from build123d import *

# Parameters (mm, degrees)
SKETCH1_W               = 8
SKETCH1_H               = 8
BOSS_EXTRUDE1_DEPTH     = 3
CUT_EXTRUDE1_DEPTH      = 12.704699911
CUT_EXTRUDE1_DEPTH_BACK = 12.704699911
CUT_EXTRUDE2_DEPTH      = 11
SKETCH4_R               = 1.8
CUT_EXTRUDE3_DEPTH      = 0.8
SKETCH5_W               = 8
SKETCH5_H               = 1
BOSS_EXTRUDE2_DEPTH     = 2
FILLET1_R               = 4
SKETCH6_W               = 0.769230769
SKETCH6_H               = 4
CUT_EXTRUDE4_DEPTH      = 0.4


with BuildPart() as part:
    # Sketch1 → Boss-Extrude1 (new body)
    with BuildSketch(Plane(origin=(0, 0, 0), x_dir=(1, 0, 0), z_dir=(0, 1, 0))):
        with Locations((4, 4)):
            Rectangle(SKETCH1_W, SKETCH1_H)
    extrude(amount=BOSS_EXTRUDE1_DEPTH)

    # Sketch2 → Cut-Extrude1 (cut, two sides: drawn at the far end of the back side and taken through both)
    with BuildSketch(Plane.XY.offset(-CUT_EXTRUDE1_DEPTH_BACK)):
        Polygon((0, 0), (0.6, 3), (0, 3), align=None)
        Polygon((8, 0), (7.4, 3), (8, 3), align=None)
    extrude(amount=CUT_EXTRUDE1_DEPTH + CUT_EXTRUDE1_DEPTH_BACK, mode=Mode.SUBTRACT)

    # Sketch3 → Cut-Extrude2 (cut)
    with BuildSketch(Plane(origin=(0, 0, 0), x_dir=(0, 0, -1), z_dir=(1, 0, 0))):
        Polygon((0, 0), (0.6, 3), (0, 3), align=None)
        Polygon((8, 3), (7.4, 3), (8, 0), align=None)
    extrude(amount=CUT_EXTRUDE2_DEPTH, mode=Mode.SUBTRACT)

    # Sketch4 → Cut-Extrude3 (cut)
    with BuildSketch(Plane.XZ):
        with Locations(Location((4, -3.75, 0), (0, 0, 270))):
            Circle(SKETCH4_R)
    extrude(amount=-CUT_EXTRUDE3_DEPTH, mode=Mode.SUBTRACT)

    # Sketch5 → Boss-Extrude2 (add)
    with BuildSketch(Plane.XZ):
        with Locations((4, -7.5)):
            Rectangle(SKETCH5_W, SKETCH5_H)
    extrude(amount=BOSS_EXTRUDE2_DEPTH)

    # Fillet1
    # the kernel refuses this fillet: 4 mm, written as the material it takes off along each edge
    with BuildSketch(Plane(origin=(8, -2, -16.660254038), x_dir=(0, 1, 0), z_dir=(0, 0, 1)), Plane(origin=(0, -2, 1.660254038), x_dir=(0, 1, 0), z_dir=(0, 0, -1))) as fillet1_piece_1:
        with BuildLine():
            CenterArc((4, 3.464101615), FILLET1_R, 180, 60)
            Line((0, 3.464101615), (-0.08, 3.464101615))
            Line((-0.08, 3.464101615), (-0.08, 0))
            Line((-0.08, 0), (0, -0.08))
            ThreePointArc((0, -0.08), (1, -0.08), (1.96, -0.069282032))
            Line((1.96, -0.069282032), (2, 0))
        make_face()
    extrude(amount=18.320508076, mode=Mode.SUBTRACT)

    # Sketch6 → Cut-Extrude4 (cut)
    with BuildSketch(Plane(origin=(0, 3, 0), x_dir=(1, 0, 0), z_dir=(0, 1, 0))):
        with Locations((4.080454652, 4.010567225)):
            Rectangle(SKETCH6_W, SKETCH6_H)
    extrude(amount=-CUT_EXTRUDE4_DEPTH, mode=Mode.SUBTRACT)


solid = part.part
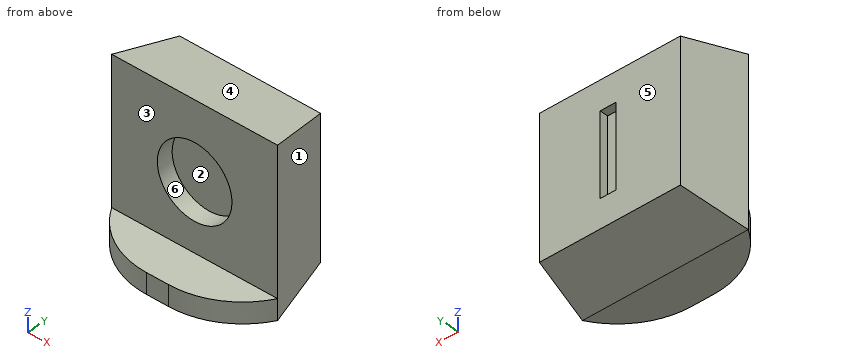
Source: CAD feature listing. Evaluate the final solid. Frame: model axes, mm. Face numbers are marked on the shaded views. A direction names the side the tool comes from. Coordinates: 2 decimals unless noted, no trailing zeros. Loops run counter-clockwise (first coordinate to the right, second up) from the corner with the lowest first, then second, coordinate; pieces in that order, holes last. Notation, with made-up numbers: (55, -4.5) - (61, -4.5) arc R32 cw to (61, 29.5) - close; hole circle Ø8 at (14.25, 51.25). An arc over 180 degrees is marked (long way). Return JSON: item names as keys, results as strings.
Q1. Access query for the marked faces 1, 2 and 3. Directions: +Z, -Z, +X, -X, +Y, -Y. A direction counts if a zero-diameter tool reaches every point of the face in a straight line with its end or side. Return the directions, or none.
Results:
{"face 1": "+Z, -Z, +X, +Y", "face 2": "-Y", "face 3": "+Z, +X, -X, -Y"}
Q2. Section A-A, the plane x = 4. Return loops of the section in (y, z).
Results:
{"outline": "(-2, -8) - (0, -8) - (3, -7.4) - (3, -6.01) - (2.6, -6.01) - (2.6, -2.01) - (3, -2.01) - (3, -0.6) - (0, 0) - (0, -1.95) - (0.8, -1.95) - (0.8, -5.55) - (0, -5.55) - (0, -7) - (-2, -7) - close"}
Q3. Section D-D, the plane x = 7. Return loops of the section in (y, z), plus the area to 3 significant figures.
Results:
{"outline": "(-1.15, -8) - (0, -8) - (3, -7.4) - (3, -0.6) - (0, 0) - (0, -7) - (-1.15, -7) - close", "area": "23.4 mm2"}
Q4. Mould query, pull axis Z, two halves, no side actions, for the marked faces 4, 5 and 6. Classes: released by +Z, released by -Z, zero draft, split by the parting line, or undercut.
Results:
{"face 4": "released by +Z", "face 5": "zero draft", "face 6": "undercut"}
Q5. Section B-B, the plane z = -3.75. Return loops of the section in (x, y).
Results:
{"outline": "(0, 0) - (2.2, 0) - (2.2, 0.8) - (5.8, 0.8) - (5.8, 0) - (8, 0) - (7.4, 3) - (4.47, 3) - (4.47, 2.6) - (3.7, 2.6) - (3.7, 3) - (0.6, 3) - close"}
Q6. Material intervals for line 1 along Y through (x, z) = (1, -3.75); line 2 along X through (y, z) = (0.65, -3.75); line 3 along Z through (x, y) = (1.5, -1.2), sorted ascending.
Results:
{"line 1": "0 to 3", "line 2": "0.13 to 2.2, 5.8 to 7.87", "line 3": "-8 to -7"}
Q7. Contact query for flat-ended pins moving along their axis: P1, Ø2, axis at x = 5, y = -1.5, coming from the +Z side; P2, Ø4, axis at x = 3.5, z = -4.5, coming from the -Y side; P3, Ø3, axis at y = 2, z = -7, coming from the -X side. Output: stop coordinate, or through.
Results:
{"P1": "z = -7", "P2": "y = 0", "P3": "x = 0.1"}
Q8. Section C-C, the plane y = 1.85. Return loops of the section in (x, z), plus the area to 3 significant figures.
Results:
{"outline": "(0.37, -7.63) - (7.63, -7.63) - (7.63, -0.37) - (0.37, -0.37) - close", "area": "52.7 mm2"}
